Geometry: final body of the model. Coordinates: model frame, mm. Face numbers are marked on the shaded views. A direction names the side the tool comes from. Give positions to 0.01 mm unless a question says otherwise; leave off trailing zeros. Write each loop counter-clockwise with the first axis right and the second up, starting at its lowest first coordinate (ties: lowest second). Pieces come first, ordered by that corner, then holes.
Q1. Cut plane C-C on x = 24. Return the cut outline in (y, z).
Q2. Line query: L1, parallel to Z at x = -57.5, y = 30.5; L2, parallel to Y at x = -56, z = -67.5; L3, parallel to Z at x = -65.5, y = 18. Output: solid intervals per line, ascending.
Q3. Draft query along Y for the marked faces 1, 2 and 3. Return one class per face: pulls with the +Y half, pulls with the -Y half, needs draft (parallel to the pull), parting line crosses it, or undercut.
Q4. Reachability of the marked faces 4, 5, 6 and 7 from +Z, -Z, +X, -X, +Y, -Y: full face, straight path, thin tool, end or side. Return the list, or none.
Q5. Pin query (flat end, axial travel): pin 1 (5.5 mm diameter, centred on x = -54.5, z = -71.5, fed in from -Y); pin 2 (5.5 mm diameter, centred on y = -2.5, z = -63, fed in from -X); pin 3 (5 mm diameter, centred on y = -24.5, z = 20.5, fed in from +X). Return the tip coordinate at first contact, or that it passes through.
Q6. Cut plane B-B on y = 0. Return the cut outline in (x, z), plus the area to 3 significant figures.
Q7. Cut plane A-A on z = 10. Return the cut outline in (x, y), plus the area to 3 significant figures.
Q8. Cut plane D-D on z = -76. Return the cut outline in (x, y).
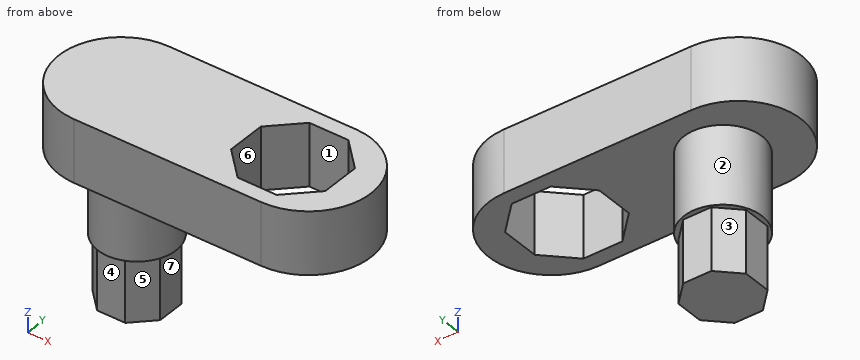
```python
from build123d import *

# Parameters (mm, degrees)
PAD_DEPTH    = 40
POCKET_DEPTH = 100
SKETCH002_R  = 25
PAD001_DEPTH = 50
PAD002_DEPTH = 40


with BuildPart() as part:
    # Sketch → Pad (new body)
    with BuildSketch(Plane.XY):
        with BuildLine():
            Line((-60, 40), (60, 40))
            ThreePointArc((60, -40), (100, 0), (60, 40))
            Line((-60, -40), (60, -40))
            ThreePointArc((-60, 40), (-100, 0), (-60, -40))
        make_face()
    extrude(amount=PAD_DEPTH)

    # Sketch001 → Pocket (cut)
    with BuildSketch(Plane(origin=(0, 0, 0), x_dir=(1, 0, 0), z_dir=(0, 0, -1))):
        Polygon((62.5, -30.17767), (80.17767, -12.5), (80.17767, 12.5), (62.5, 30.17767), (37.5, 30.17767), (19.82233, 12.5), (19.82233, -12.5), (37.5, -30.17767), align=None)
    extrude(amount=-POCKET_DEPTH, mode=Mode.SUBTRACT)

    # Sketch002 → Pad001 (join)
    with BuildSketch(Plane(origin=(0, 0, 0), x_dir=(1, 0, 0), z_dir=(0, 0, -1))):
        with Locations((-50, 0)):
            Circle(SKETCH002_R)
    extrude(amount=PAD001_DEPTH)

    # Sketch003 → Pad002 (join)
    with BuildSketch(Plane(origin=(0, 0, -50), x_dir=(1, 0, 0), z_dir=(0, 0, -1))):
        Polygon((-41, -21.727922), (-28.272078, -9), (-28.272078, 9), (-41, 21.727922), (-59, 21.727922), (-71.727922, 9), (-71.727922, -9), (-59, -21.727922), align=None)
    extrude(amount=PAD002_DEPTH)


solid = part.part
```
Data:
1. outline: (-40, 0) - (-16.68, 0) - (-16.68, 40) - (-40, 40) - close; (16.68, 0) - (40, 0) - (40, 40) - (16.68, 40) - close
2. L1: z = 0 to 40
2. L2: y = -21.73 to 21.73
2. L3: z = -50 to 40
3. face 1: undercut
3. face 2: parting line crosses it
3. face 3: pulls with the +Y half
4. face 4: -Z, +X, -X, -Y
4. face 5: -Z, +X, -Y
4. face 6: +Z, -Z
4. face 7: -Z, +X, +Y, -Y
5. pin 1: stops at y = -21.73
5. pin 2: stops at x = -71.73
5. pin 3: stops at x = 93.41
6. outline: (-100, 0) - (-75, 0) - (-75, -50) - (-71.73, -50) - (-71.73, -90) - (-28.27, -90) - (-28.27, -50) - (-25, -50) - (-25, 0) - (19.82, 0) - (19.82, 40) - (-100, 40) - close; (80.18, 0) - (100, 0) - (100, 40) - (80.18, 40) - close
6. area: 9,820 mm2
7. outline: (-60, -40) - (60, -40) arc R40 ccw to (60, 40) - (-60, 40) arc R40 ccw to start; hole (19.82, -12.5) - (37.5, -30.18) - (62.5, -30.18) - (80.18, -12.5) - (80.18, 12.5) - (62.5, 30.18) - (37.5, 30.18) - (19.82, 12.5) - close
7. area: 11,600 mm2
8. outline: (-71.73, -9) - (-59, -21.73) - (-41, -21.73) - (-28.27, -9) - (-28.27, 9) - (-41, 21.73) - (-59, 21.73) - (-71.73, 9) - close
